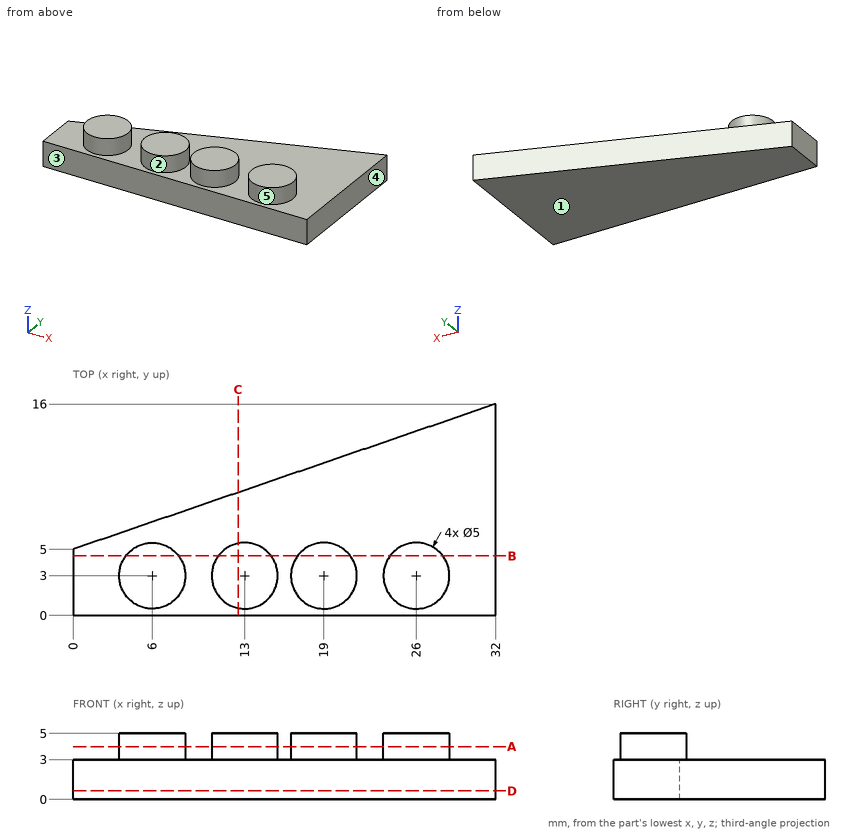
Input: dimensioned drawing with shaded views. Units: mm. Origin: part minimum x, y, z. A direction names the side the tool comes from. Give positions to 0.01 mm unless a question says otherwise; leave off trailing zeros. Write each loop counter-clockwise with the first axis right and the second up, starting at its lowest first coordinate (ties: lowest second). Pieces come first, ordered by that corner, then holes. Notation, with made-up numbers: (-24, -23.75) -> (-9, -23.75) arc R23 cw to (-9, -12.75) -> close; hole circle Ø8 at (6, -31). An arc over 180 degrees is marked (long way). Return JSON: item names as keys, results as strings. Group by question number.
1. Section B-B, the plane y = 4.5. Output: boundary loops of the cut face in (x, z), then the cut area to 3 significant figures.
2. Section D-D, the plane z = 0.65. Output: boundary loops of the cut face in (x, y).
3. Material intervals for line 1 (X direction, y = 2.5, z = 4.1); line 2 (Z direction, x = 18, y = 7); line 3 (Y direction, x = 5, z = 2.4), sorted ascending. Write a range as from..to.
4. Pin query (flat end, axial travel): pin 1 Ø3 at (x, z) = (26.5, 1) entering from +Y (3 decimals); pin 2 Ø1.5 at (x, z) = (24, 3.5) entering from +Y; pin 3 Ø5 at (x, y) = (8.5, 5) entering from +Z. Return the tip coordinate at first contact, or that it passes through.
5. Section A-A, the plane z = 4. Output: boundary loops of the cut face in (x, y), then the cut area to 3 significant figures.
6. Access query for the marked faces 1 and 2. Directions: +Z, -Z, +X, -X, +Y, -Y. A direction counts if a zero-diameter tool reaches every point of the face in a straight line with its end or side. Return the directions, or none.
7. Section C-C, the plane x = 12.5. Output: boundary loops of the cut face in (y, z).
8. Mould query, pull axis X, two halves, no side actions, for the marked faces 3, 4 and 5. Classes: +X half, -X half, draft (parallel to the pull), parting line (faces both ways), or undercut.
Determined:
{
 "1": {"outline": "(0, 0) -> (32, 0) -> (32, 3) -> (28, 3) -> (28, 5) -> (24, 5) -> (24, 3) -> (21, 3) -> (21, 5) -> (17, 5) -> (17, 3) -> (15, 3) -> (15, 5) -> (11, 5) -> (11, 3) -> (8, 3) -> (8, 5) -> (4, 5) -> (4, 3) -> (0, 3) -> close", "area": "128 mm2"},
 "2": {"outline": "(0, 0) -> (32, 0) -> (32, 16) -> (0, 5) -> close"},
 "3": {"line 1": "x = 3.55..8.45, 10.55..15.45, 16.55..21.45, 23.55..28.45", "line 2": "z = 0..3", "line 3": "y = 0..6.72"},
 "4": {"pin 1": "stops at y = 14.625", "pin 2": "stops at y = 13.44", "pin 3": "stops at z = 5"},
 "5": {"outline": "circle Ø5 at (6, 3); circle Ø5 at (13, 3); circle Ø5 at (19, 3); circle Ø5 at (26, 3)", "area": "78.5 mm2"},
 "6": {"face 1": "-Z, +X, -X, +Y, -Y", "face 2": "+Z"},
 "7": {"outline": "(0, 0) -> (9.3, 0) -> (9.3, 3) -> (5.45, 3) -> (5.45, 5) -> (0.55, 5) -> (0.55, 3) -> (0, 3) -> close"},
 "8": {"face 3": "draft", "face 4": "+X half", "face 5": "undercut"}
}
